```python
from build123d import *

# Parameters (mm, degrees)
SKETCH_1_R      = 6.4
EXTRUDE_1_DEPTH = 22
SKETCH_2_R      = 11.1
SKETCH_2_R_2    = 1.6
EXTRUDE_3_DEPTH = 2
SKETCH_3_R      = 2.5
EXTRUDE_4_DEPTH = 1.5


with BuildPart() as part:
    # 草图1 → 凸台-拉伸1 (new body)
    with BuildSketch(Plane(origin=(0, 0, 0), x_dir=(1, 0, 0), z_dir=(0, 1, 0))):
        with Locations(Location((0, 0, 0), (0, 0, 270))):
            Circle(SKETCH_1_R)
    extrude(amount=EXTRUDE_1_DEPTH)

    # 草图2 → 凸台-拉伸3 (add)
    with BuildSketch(Plane(origin=(0, 22, 0), x_dir=(1, 0, 0), z_dir=(0, 1, 0))):
        with Locations(Location((0, 0, 0), (0, 0, 270))):
            Circle(SKETCH_2_R)
        with Locations(Location((0, 8.75, 0), (0, 0, 270))):
            Circle(SKETCH_2_R_2, mode=Mode.SUBTRACT)
        with Locations(Location((7.577722283, -4.375, 0), (0, 0, 270))):
            Circle(SKETCH_2_R_2, mode=Mode.SUBTRACT)
        with Locations(Location((-7.577722283, -4.375, 0), (0, 0, 270))):
            Circle(SKETCH_2_R_2, mode=Mode.SUBTRACT)
    extrude(amount=EXTRUDE_3_DEPTH)

    # 草图3 → 凸台-拉伸4 (add)
    with BuildSketch(Plane(origin=(0, 24, 0), x_dir=(1, 0, 0), z_dir=(0, 1, 0))):
        with Locations(Location((0, 0, 0), (0, 0, 270))):
            Circle(SKETCH_3_R)
    extrude(amount=EXTRUDE_4_DEPTH)


solid = part.part
```
The model under review builds one solid part; all positions refer to its coordinate system, in mm. A direction names the side the tool comes from. Give positions to 0.01 mm unless a question says otherwise; leave off trailing zeros. Write each loop counter-clockwise with the first axis right and the second up, starting at its lowest first coordinate (ties: lowest second). Pieces come first, ordered by that corner, then holes. Notation, with made-up numbers: (52.25, 34) - (99.25, 34) arc R15 ccw to (99.25, 51) - close; hole circle Ø6 at (34.5, 19.25). An arc over 180 degrees is marked (long way). Answer in a Markdown table with one row per item. Add a question column.
1. Draft analysis for pull direction X (two halves, no side actions). For faces 1 (the cylindrical face through (-2.44, 24.74, -0.54)), 2 (the flat face through (3, 24, 0)), 3 (the cylindrical face through (0.07, 22.99, -10.35)), state which applies: +X half, -X half, draft (parallel to the pull), parting line (faces both ways), or undercut.
2. We need section A-A on x = 0. Write out the cut boundary in (y, z), then the cut area to 3 significant figures.
3. Wall thickness on line 1 along Y through (x, z) = (1, 5.25); line 2 along Y through (x, z) = (8, -4.25); line 3 along X through (y, z) = (22.5, -8.75): over which ranges is each line inside the solid? List them lowest first. Write a range as [from, to].
4. Insertion check: P1, Ø1, axis at x = -1, z = 6, coming from the +Y side; P2, Ø3, axis at x = 7.58, z = 4.38, coming from the +Y side; P3, Ø8, axis at x = -2.5, y = 15.5, coming from the -Z side; P4, Ø8, axis at y = 7, z = 4.5, coming from the +X side. Each pin has a flat end and moves straight along its axis. Give the tip position at first contact, or say it passes through.
5. Tool access review of faces 4 (the cylindrical face through (-3.89, 10.85, -5.08)), 5 (the cylindrical face through (-5.99, 22.99, 4.17)): name each direction out of +Z, -Z, +X, -X, +Y, -Y from which nothing blocks a thin tool from reaching the whole face with its end or side.
6. We need section C-C on z = -8.75. Write out the cut boundary in (x, y), then the cut area to 3 significant figures.
7. We need section D-D on y = 11.75. Write out the cut boundary in (x, z), then the cut area to 3 significant figures.
8. We need section B-B on z = 0. Write out the cut boundary in (x, y).
Ans:
| question | item | result |
|---|---|---|
| 1 | face 1 | parting line |
| 1 | face 2 | draft |
| 1 | face 3 | undercut |
| 2 | outline | (0, -6.4) - (22, -6.4) - (22, -7.15) - (24, -7.15) - (24, -2.5) - (25.5, -2.5) - (25.5, 2.5) - (24, 2.5) - (24, 11.1) - (22, 11.1) - (22, 6.4) - (0, 6.4) - close; (22, -11.1) - (24, -11.1) - (24, -10.35) - (22, -10.35) - close |
| 2 | area | 327 mm^2 |
| 3 | line 1 | y = [0, 24] |
| 3 | line 2 | y = [22, 24] |
| 3 | line 3 | x = [-6.83, -1.6], [1.6, 6.83] |
| 4 | P1 | stops at y = 24 |
| 4 | P2 | passes through |
| 4 | P3 | stops at z = -6.4 |
| 4 | P4 | stops at x = 6.38 |
| 5 | face 4 | -Y |
| 5 | face 5 | +Y, -Y |
| 6 | outline | (-6.83, 22) - (-1.6, 22) - (-1.6, 24) - (-6.83, 24) - close; (1.6, 22) - (6.83, 22) - (6.83, 24) - (1.6, 24) - close |
| 6 | area | 20.9 mm^2 |
| 7 | outline | circle Ø12.8 at (0, 0) |
| 7 | area | 129 mm^2 |
| 8 | outline | (-11.1, 22) - (-6.4, 22) - (-6.4, 0) - (6.4, 0) - (6.4, 22) - (11.1, 22) - (11.1, 24) - (2.5, 24) - (2.5, 25.5) - (-2.5, 25.5) - (-2.5, 24) - (-11.1, 24) - close |
